Geometry: final body of the model. Coordinates: model frame, mm. A direction names the side the tool comes from. Give positions to 0.01 mm unless a question says otherwise; leave off trailing zeros. Write each loop counter-clockwise with the first axis right and the second up, starting at its lowest first coordinate (ties: lowest second). Pieces come first, ordered by that corner, then holes.
from build123d import *
from OCP.BRepFilletAPI import BRepFilletAPI_MakeChamfer

# Parameters (mm, degrees)
SKETCH1_W           = 86
SKETCH1_H           = 74
BOSS_EXTRUDE1_DEPTH = 25
SKETCH3_W           = 82
SKETCH3_H           = 70
CUT_EXTRUDE1_DEPTH  = 23
SKETCH4_W           = 8
SKETCH4_H           = 37.5
SKETCH4_W_2         = 1.4
BOSS_EXTRUDE2_DEPTH = 5
SKETCH5_W           = 3
SKETCH5_H           = 8
SKETCH5_W_2         = 1
SKETCH5_H_2         = 4
CUT_EXTRUDE2_DEPTH  = 2
SKETCH6_R           = 1
CUT_EXTRUDE3_DEPTH  = 5
SKETCH7_W           = 4
SKETCH7_H           = 35
CUT_EXTRUDE4_DEPTH  = 5
SKETCH9_W           = 5
SKETCH9_H           = 32.5
SKETCH9_W_2         = 6
BOSS_EXTRUDE3_DEPTH = 3
SKETCH10_R          = 0.9
CUT_EXTRUDE6_DEPTH  = 4
FILLET1_R           = 2
SKETCH13_R          = 2
SKETCH13_W          = 13
SKETCH13_H          = 3.4
CUT_EXTRUDE9_DEPTH  = 4
CHAMFER1_SIZE       = 1.4
CHAMFER1_SIZE2      = 2.240468341
SKETCH14_R          = 0.8
CUT_EXTRUDE10_DEPTH = 76
SKETCH15_R          = 1.5
CUT_EXTRUDE11_DEPTH = 0.6
CUT_EXTRUDE12_START = -0.6
SKETCH16_R          = 1.5
CUT_EXTRUDE12_DEPTH = 0.6
SKETCH20_W          = 11
SKETCH20_H          = 1.4
BOSS_EXTRUDE6_DEPTH = 5
SKETCH21_W          = 13
SKETCH21_H          = 16
CUT_EXTRUDE13_DEPTH = 10
SKETCH22_W          = 3
SKETCH22_H          = 12
BOSS_EXTRUDE7_DEPTH = 12
CUT_EXTRUDE14_DEPTH = 3
SKETCH24_R          = 3.5
CUT_EXTRUDE15_DEPTH = 3
FILLET2_R           = 3
SKETCH27_W          = 3.6
SKETCH27_H          = 10
CUT_EXTRUDE16_DEPTH = 3
FILLET3_R           = 1.8
FILLET4_R           = 1
FILLET5_R           = 2
SKETCH28_W          = 8
SKETCH28_H          = 2
CUT_EXTRUDE17_DEPTH = 0.4
SKETCH29_W          = 8
SKETCH29_H          = 2
CUT_EXTRUDE18_DEPTH = 0.4
FILLET6_R           = 0.4


with BuildPart() as part:
    # Sketch1 → Boss-Extrude1 (new body)
    with BuildSketch(Plane.XY):
        with Locations((43, 37)):
            Rectangle(SKETCH1_W, SKETCH1_H)
    extrude(amount=BOSS_EXTRUDE1_DEPTH)

    # Sketch3 → Cut-Extrude1 (cut)
    with BuildSketch(Plane.XY.offset(25)):
        with Locations((43, 37)):
            Rectangle(SKETCH3_W, SKETCH3_H)
    extrude(amount=-CUT_EXTRUDE1_DEPTH, mode=Mode.SUBTRACT)

    # Sketch4 → Boss-Extrude2 (add)
    with BuildSketch(Plane.XY.offset(2)):
        with Locations((80, 53.25)):
            Rectangle(SKETCH4_W, SKETCH4_H)
        with Locations((12.3, 53.25)):
            Rectangle(SKETCH4_W_2, SKETCH4_H)
    extrude(amount=BOSS_EXTRUDE2_DEPTH)

    # Sketch5 → Cut-Extrude2 (cut)
    with BuildSketch(Plane.XY.offset(7)):
        with Locations((77.5, 58)):
            Rectangle(SKETCH5_W, SKETCH5_H)
        with Locations((76.5, 43.5)):
            Rectangle(SKETCH5_W_2, SKETCH5_H_2)
    extrude(amount=-CUT_EXTRUDE2_DEPTH, mode=Mode.SUBTRACT)

    # Sketch6 → Cut-Extrude3 (cut)
    with BuildSketch(Plane.XY.offset(7)):
        with Locations((80, 67.25)):
            Circle(SKETCH6_R)
        with Locations((80, 39.25)):
            Circle(SKETCH6_R)
    extrude(amount=-CUT_EXTRUDE3_DEPTH, mode=Mode.SUBTRACT)

    # Sketch7 → Cut-Extrude4 (cut)
    with BuildSketch(Plane(origin=(2, 0, 0), x_dir=(0, 0, -1), z_dir=(1, 0, 0))):
        with Locations((-4.4, 53.35)):
            Rectangle(SKETCH7_W, SKETCH7_H)
    extrude(amount=-CUT_EXTRUDE4_DEPTH, mode=Mode.SUBTRACT)

    # Sketch9 → Boss-Extrude3 (add)
    with BuildSketch(Plane.XY.offset(2)):
        with Locations((81.5, 18.25)):
            Rectangle(SKETCH9_W, SKETCH9_H)
        with Locations((59, 18.25)):
            Rectangle(SKETCH9_W_2, SKETCH9_H)
        with Locations((4.5, 18.25)):
            Rectangle(SKETCH9_W, SKETCH9_H)
        with Locations((27, 18.25)):
            Rectangle(SKETCH9_W_2, SKETCH9_H)
    extrude(amount=BOSS_EXTRUDE3_DEPTH)

    # Sketch10 → Cut-Extrude6 (cut)
    with BuildSketch(Plane.XY.offset(5)):
        with Locations((59, 13.5)):
            Circle(SKETCH10_R)
        with Locations((27, 16.5)):
            Circle(SKETCH10_R)
    extrude(amount=-CUT_EXTRUDE6_DEPTH, mode=Mode.SUBTRACT)

    # Fillet1
    fillet1_edges = [part.edges().sort_by_distance(p)[0] for p in [
        (0, 74, 12.5),
        (86, 74, 12.5),
        (86, 0, 12.5),
        (0, 0, 12.5),
    ]]
    fillet(fillet1_edges, radius=FILLET1_R)

    # Sketch13 → Cut-Extrude9 (cut)
    with BuildSketch(Plane(origin=(0, 72, 0), x_dir=(-1, 0, 0), z_dir=(0, -1, 0))):
        with Locations(Location((-37, -9.8, 0), (0, 0, 90))):
            Circle(SKETCH13_R)
        with Locations(Location((-46, -9.8, 0), (0, 0, 90))):
            Circle(SKETCH13_R)
        with Locations((-22.5, -9.3)):
            Rectangle(SKETCH13_W, SKETCH13_H)
    extrude(amount=-CUT_EXTRUDE9_DEPTH, mode=Mode.SUBTRACT)

    # Chamfer1: one chamfer whose edges measure the first distance from different faces: ONE call of the kernel's chamfer builder (chamfer() names one face for all edges)
    chamfer1_edges_1 = [part.edges().sort_by_distance(p)[0] for p in [
        (16, 74, 9.3),
    ]]
    chamfer1_side_1 = [part.faces().sort_by_distance(p)[0] for p in [
        (16, 73, 9.3),
    ]]
    chamfer1_edges_2 = [part.edges().sort_by_distance(p)[0] for p in [
        (29, 74, 9.3),
    ]]
    chamfer1_side_2 = [part.faces().sort_by_distance(p)[0] for p in [
        (29, 73, 9.3),
    ]]
    chamfer1_edges_3 = [part.edges().sort_by_distance(p)[0] for p in [
        (37, 74, 11.8),
    ]]
    chamfer1_side_3 = [part.faces().sort_by_distance(p)[0] for p in [
        (37, 73, 11.8),
    ]]
    chamfer1_edges_4 = [part.edges().sort_by_distance(p)[0] for p in [
        (46, 74, 11.8),
    ]]
    chamfer1_side_4 = [part.faces().sort_by_distance(p)[0] for p in [
        (46, 73, 11.8),
    ]]
    chamfer1 = BRepFilletAPI_MakeChamfer(part.part.solid().wrapped)
    for e in chamfer1_edges_1:
        chamfer1.Add(CHAMFER1_SIZE, CHAMFER1_SIZE2, e.wrapped, chamfer1_side_1[0].wrapped)  # the first distance lies on this face
    for e in chamfer1_edges_2:
        chamfer1.Add(CHAMFER1_SIZE, CHAMFER1_SIZE2, e.wrapped, chamfer1_side_2[0].wrapped)  # the first distance lies on this face
    for e in chamfer1_edges_3:
        chamfer1.Add(CHAMFER1_SIZE, CHAMFER1_SIZE2, e.wrapped, chamfer1_side_3[0].wrapped)  # the first distance lies on this face
    for e in chamfer1_edges_4:
        chamfer1.Add(CHAMFER1_SIZE, CHAMFER1_SIZE2, e.wrapped, chamfer1_side_4[0].wrapped)  # the first distance lies on this face
    add(Compound.cast(chamfer1.Shape()), mode=Mode.REPLACE)

    # Sketch14 → Cut-Extrude10 (cut)
    with BuildSketch(Plane(origin=(0, 0, 0), x_dir=(-1, 0, 0), z_dir=(0, -1, 0))):
        with Locations(Location((-10, -23, 0), (0, 0, 90))):
            Circle(SKETCH14_R)
        with Locations(Location((-76, -23, 0), (0, 0, 90))):
            Circle(SKETCH14_R)
    extrude(amount=-CUT_EXTRUDE10_DEPTH, mode=Mode.SUBTRACT)

    # Sketch15 → Cut-Extrude11 (cut)
    with BuildSketch(Plane(origin=(0, 0, 0), x_dir=(-1, 0, 0), z_dir=(0, -1, 0))):
        with Locations(Location((-10, -23, 0), (0, 0, 90))):
            Circle(SKETCH15_R)
        with Locations(Location((-76, -23, 0), (0, 0, 90))):
            Circle(SKETCH15_R)
    extrude(amount=-CUT_EXTRUDE11_DEPTH, mode=Mode.SUBTRACT)

    # Sketch16 → Cut-Extrude12 (cut)
    with BuildSketch(Plane(origin=(0, 74, 0), x_dir=(1, 0, 0), z_dir=(0, 1, 0)).offset(CUT_EXTRUDE12_START)):
        with Locations(Location((76, -23, 0), (0, 0, 90))):
            Circle(SKETCH16_R)
        with Locations(Location((10, -23, 0), (0, 0, 90))):
            Circle(SKETCH16_R)
    extrude(amount=CUT_EXTRUDE12_DEPTH, mode=Mode.SUBTRACT)

    # Sketch20 → Boss-Extrude6 (add)
    with BuildSketch(Plane.XY.offset(2)):
        with Locations((7.5, 33.8)):
            Rectangle(SKETCH20_W, SKETCH20_H)
    extrude(amount=BOSS_EXTRUDE6_DEPTH)

    # Sketch21 → Cut-Extrude13 (cut)
    with BuildSketch(Plane(origin=(2, 0, 0), x_dir=(0, 0, -1), z_dir=(1, 0, 0))):
        with Locations((-13.1, 14)):
            Rectangle(SKETCH21_W, SKETCH21_H)
    extrude(amount=-CUT_EXTRUDE13_DEPTH, mode=Mode.SUBTRACT)

    # Sketch22 → Boss-Extrude7 (add)
    with BuildSketch(Plane.XY.offset(5)):
        with Locations((82.5, 18.25)):
            Rectangle(SKETCH22_W, SKETCH22_H)
    extrude(amount=BOSS_EXTRUDE7_DEPTH)

    # Sketch23 → Cut-Extrude14 (cut)
    with BuildSketch(Plane.ZY.offset(-81)):
        Polygon((6.7, 15.767393842), (11, 13.284787685), (15.3, 15.767393842), (15.3, 20.732606158), (11, 23.215212315), (6.7, 20.732606158), align=None)
    extrude(amount=-CUT_EXTRUDE14_DEPTH, mode=Mode.SUBTRACT)

    # Sketch24 → Cut-Extrude15 (cut)
    with BuildSketch(Plane.ZY.offset(-84)):
        with Locations((11, 18.25)):
            Circle(SKETCH24_R)
    extrude(amount=-CUT_EXTRUDE15_DEPTH, mode=Mode.SUBTRACT)

    # Fillet2
    fillet2_edges = [part.edges().sort_by_distance(p)[0] for p in [
        (82.5, 24.25, 5),
        (82.5, 12.25, 5),
        (82.5, 24.25, 17),
        (82.5, 12.25, 17),
    ]]
    fillet(fillet2_edges, radius=FILLET2_R)

    # Sketch27 → Cut-Extrude16 (cut)
    with BuildSketch(Plane.ZY.offset(-84)):
        with Locations((9.8, 46.5)):
            Rectangle(SKETCH27_W, SKETCH27_H)
    extrude(amount=-CUT_EXTRUDE16_DEPTH, mode=Mode.SUBTRACT)

    # Fillet3
    fillet3_edges = [part.edges().sort_by_distance(p)[0] for p in [
        (85, 41.5, 8),
        (85, 41.5, 11.6),
        (85, 51.5, 8),
        (85, 51.5, 11.6),
    ]]
    fillet(fillet3_edges, radius=FILLET3_R - 0.0001)  # a hair under: the kernel refuses the full size

    # Fillet4
    fillet4_edges = [part.edges().sort_by_distance(p)[0] for p in [
        (86, 46.5, 8),
        (86, 46.5, 11.6),
        (86, 42.027178505, 8.527178505),
        (86, 42.027178505, 11.072821495),
        (86, 50.972821495, 8.527178505),
        (86, 50.972821495, 11.072821495),
    ]]
    fillet(fillet4_edges, radius=FILLET4_R)

    # Fillet5
    fillet5_edges = [part.edges().sort_by_distance(p)[0] for p in [
        (84, 5.625, 5),
        (84, 11.371320344, 5.878679656),
        (84, 12.25, 11),
        (84, 13.128679656, 16.121320344),
        (84, 30.875, 5),
        (84, 25.128679656, 5.878679656),
        (84, 24.25, 11),
        (84, 23.371320344, 16.121320344),
        (84, 18.25, 17),
    ]]
    fillet(fillet5_edges, radius=FILLET5_R)

    # Sketch28 → Cut-Extrude17 (cut)
    with BuildSketch(Plane(origin=(0, 0, 0), x_dir=(-1, 0, 0), z_dir=(0, -1, 0))):
        with Locations((-11, -4)):
            Rectangle(SKETCH28_W, SKETCH28_H)
        with Locations((-75, -4)):
            Rectangle(SKETCH28_W, SKETCH28_H)
    extrude(amount=-CUT_EXTRUDE17_DEPTH, mode=Mode.SUBTRACT)

    # Sketch29 → Cut-Extrude18 (cut)
    with BuildSketch(Plane(origin=(0, 74, 0), x_dir=(1, 0, 0), z_dir=(0, 1, 0))):
        with Locations((75, -4)):
            Rectangle(SKETCH29_W, SKETCH29_H)
        with Locations((11, -4)):
            Rectangle(SKETCH29_W, SKETCH29_H)
    extrude(amount=-CUT_EXTRUDE18_DEPTH, mode=Mode.SUBTRACT)

    # Fillet6
    fillet6_edges = [part.edges().sort_by_distance(p)[0] for p in [
        (75, 0.4, 5),
        (75, 0.4, 3),
        (11, 0.4, 3),
        (11, 0.4, 5),
        (11, 73.6, 5),
        (11, 73.6, 3),
        (75, 73.6, 3),
        (75, 73.6, 5),
    ]]
    fillet(fillet6_edges, radius=FILLET6_R - 0.0001)  # a hair under: the kernel refuses the full size


solid = part.part
Q1. Ray query, line 1 along X through (y, z) = (67.25, 4.55); line 2 along Y through (x, z) = (67, 18.75); line 3 along X through (y, z) = (69.5, 20.5). Return the intervals inside material, ascending.
Filled sheet:
line 1: x = 11.6 to 13, 76 to 79, 81 to 86
line 2: y = 0 to 2, 72 to 74
line 3: x = 0 to 2, 84 to 86
Q2. Access query for faces 1 (the cylindrical face through (84.507, 42.041, 8.513)), 2 (the flat face through (80, 54, 7)), 3 (the cylindrical face through (74.513, 73.696, 23.195)), 4 (the flat face through (1, 53, 6.4)). Directions: +Z, -Z, +X, -X, +Y, -Y. A direction counts if a zero-diameter tool reaches every point of the face in a straight line with its end or side. Return the directions, or none.
Filled sheet:
face 1: +X
face 2: +Z
face 3: +Y
face 4: -X
Q3. Section B-B on y = 61. Output: boundary loops of the cut face in (x, z), plus the area to 3 significant figures.
Filled sheet:
outline: (0, 0) - (86, 0) - (86, 25) - (84, 25) - (84, 7) - (79, 7) - (79, 5) - (76, 5) - (76, 2) - (13, 2) - (13, 7) - (11.6, 7) - (11.6, 2) - (2, 2) - (2, 2.4) - (0, 2.4) - close; (0, 6.4) - (2, 6.4) - (2, 25) - (0, 25) - close
area: 297 mm2
Q4. Section A-A on x = 37. Output: boundary loops of the cut face in (y, z).
Filled sheet:
outline: (0, 0) - (74, 0) - (74, 5.56) - (72.6, 7.8) - (72, 7.8) - (72, 2) - (2, 2) - (2, 25) - (0, 25) - close; (72, 11.8) - (72.6, 11.8) - (74, 14.04) - (74, 25) - (72, 25) - close
Q5. Pin query (flat end, axial travel): P1, Ø1, axis at x = 75.5, z = 4, coming from the -Y side; P2, Ø1.8, axis at x = 59.5, y = 15, coming from the +Z side. Return the tip coordinate at first contact, or that it passes through.
Filled sheet:
P1: stops at y = 0.4
P2: stops at z = 5
Q6. Section D-D on y = 5. Output: boundary loops of the cut face in (x, z).
Filled sheet:
outline: (0, 0) - (86, 0) - (86, 25) - (84, 25) - (84, 7) arc R2 cw to (82, 5) - (79, 5) - (79, 2) - (62, 2) - (62, 5) - (56, 5) - (56, 2) - (30, 2) - (30, 5) - (24, 5) - (24, 2) - (7, 2) - (7, 5) - (2, 5) - (2, 25) - (0, 25) - close
Q7. Pull-direction query (Y, two-part tool) for faces 5 (the flat face through (10, 73.4, 22)), 6 (the flat face through (59, 34.5, 3)), 7 (the flat face through (42, 0, 12)); classes: released by +Y, released by -Y, zero draft, split by the parting line, or undercut.
Filled sheet:
face 5: released by +Y
face 6: undercut
face 7: released by -Y
Q8. Section C-C on x = 52.5. Output: boundary loops of the cut face in (y, z), plus the area to 3 significant figures.
Filled sheet:
outline: (0, 0) - (74, 0) - (74, 25) - (72, 25) - (72, 2) - (2, 2) - (2, 25) - (0, 25) - close
area: 240 mm2
